Design review of the part shown in the three views and the two pictorial views. Dimensions are in mm from the part's minimum x, y and z. A direction names the side the tool comes from. Give positions to 0.01 mm unless a question says otherwise; leave off trailing zeros. Write each loop counter-clockwise with the first axis right and the second up, starting at its lowest first coordinate (ties: lowest second). Pieces come first, ordered by that corner, then holes.
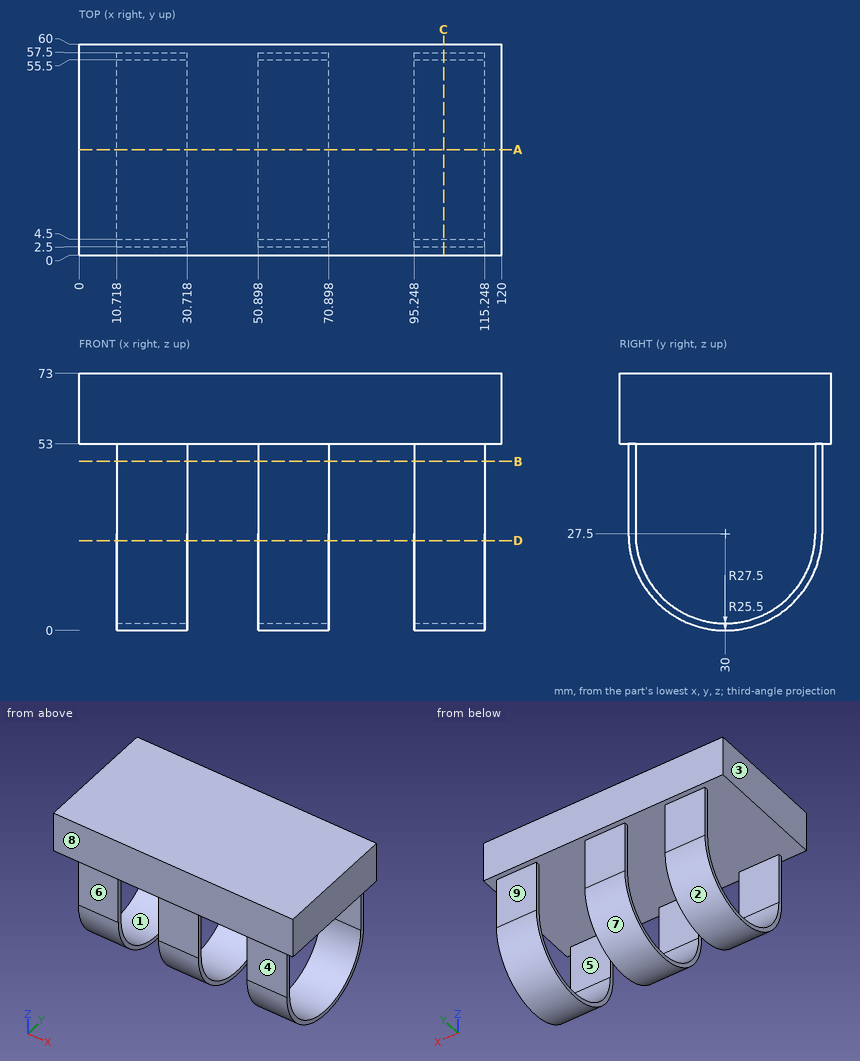
(1) Consider section B-B, the plane z = 48. Give the boundary of the cut face in (x, y), then the cut area to 3 significant figures.
Resolved:
outline: (10.72, 2.5) - (30.72, 2.5) - (30.72, 4.5) - (10.72, 4.5) - close; (10.72, 55.5) - (30.72, 55.5) - (30.72, 57.5) - (10.72, 57.5) - close; (50.9, 2.5) - (70.9, 2.5) - (70.9, 4.5) - (50.9, 4.5) - close; (50.9, 55.5) - (70.9, 55.5) - (70.9, 57.5) - (50.9, 57.5) - close; (95.25, 2.5) - (115.25, 2.5) - (115.25, 4.5) - (95.25, 4.5) - close; (95.25, 55.5) - (115.25, 55.5) - (115.25, 57.5) - (95.25, 57.5) - close
area: 240 mm2
(2) To check wall thickness, follow L1, parallel to Y at x = 66.5, z = 43.5; L2, parallel to Z at x = 32, y = 9.5; L3, parallel to Z at x = 97.5, y = 42.5 (1 decimal). State the ranges of each line that lie inside material, in increasing order.
Resolved:
L1: y = 2.5 to 4.5, 55.5 to 57.5
L2: z = 53 to 73
L3: z = 3 to 5.3, 53 to 73
(3) Clearance check with flat-ended pins moving along their axes: P1, Ø6, axis at x = 61.5, z = 45, coming from the -Y side; P2, Ø3, axis at x = 55, y = 52.5, coming from the -Z side (1 decimal); P3, Ø3, axis at x = 52.5, y = 17, coming from the -Z side; P4, Ø1.5, axis at y = 54, z = 40.5, coming from the -X side. State where each tip first meets the part, or that it passes through.
Resolved:
P1: stops at y = 2.5
P2: stops at z = 9.7
P3: stops at z = 2.52
P4: passes through
(4) Tool access review of the marked faces 5, 6, 7, 8 and 9: name each direction out of +Z, -Z, +X, -X, +Y, -Y from which nothing blocks a thin tool from reaching the whole face with its end or side.
Resolved:
face 5: +X, -X
face 6: -Z, +X, -X, -Y
face 7: -Z, +X, -X
face 8: +Z, -Z, +X, -X, -Y
face 9: -Z, +X, -X, +Y
(5) Consider section D-D, the plane z = 25.5. Give the boundary of the cut face in (x, y).
Resolved:
outline: (10.72, 2.57) - (30.72, 2.57) - (30.72, 4.58) - (10.72, 4.58) - close; (10.72, 55.42) - (30.72, 55.42) - (30.72, 57.43) - (10.72, 57.43) - close; (50.9, 2.57) - (70.9, 2.57) - (70.9, 4.58) - (50.9, 4.58) - close; (50.9, 55.42) - (70.9, 55.42) - (70.9, 57.43) - (50.9, 57.43) - close; (95.25, 2.57) - (115.25, 2.57) - (115.25, 4.58) - (95.25, 4.58) - close; (95.25, 55.42) - (115.25, 55.42) - (115.25, 57.43) - (95.25, 57.43) - close
(6) Consider section A-A, the plane y = 30. Give the boundary of the cut face in (x, z).
Resolved:
outline: (0, 53) - (120, 53) - (120, 73) - (0, 73) - close; (10.72, 0) - (30.72, 0) - (30.72, 2) - (10.72, 2) - close; (50.9, 0) - (70.9, 0) - (70.9, 2) - (50.9, 2) - close; (95.25, 0) - (115.25, 0) - (115.25, 2) - (95.25, 2) - close
(7) Consider section C-C, the plane x = 103.5. Give the boundary of the cut face in (y, z).
Resolved:
outline: (0, 53) - (2.5, 53) - (2.5, 27.5) arc R27.5 ccw to (57.5, 27.5) - (57.5, 53) - (60, 53) - (60, 73) - (0, 73) - close; hole (4.5, 27.5) arc R25.5 ccw to (55.5, 27.5) - (55.5, 53) - (4.5, 53) - close
(8) Mouldability with a two-part tool opening along Y and no side actions: class the marked faces 1, 2, 3 and 4 as pulls with the +Y half, pulls with the -Y half, needs draft (parallel to the pull), parting line crosses it, or undercut.
Resolved:
face 1: undercut
face 2: parting line crosses it
face 3: needs draft
face 4: pulls with the -Y half
